Can you work these out from the model? Positions are in its coordinate system, mm. A direction names the side the tool comes from. Coordinates: 2 decimals unless noted, no trailing zeros. Loops run counter-clockwise (first coordinate to the right, second up) from the corner with the lowest first, then second, coordinate; pieces in that order, holes last.
```python
from build123d import *

# Parameters (mm, degrees)
F2_R     = 1.5875
F3_DEPTH = 11.1125
F4_R     = 4.7625
F5_DEPTH = 9.525


with BuildPart() as f1:
    # F0 (on Front) → F1 (revolve)
    with BuildSketch(Plane.XZ):
        with BuildLine():
            Line((0, 63.5), (0, 0))
            Line((0, 0), (5.658861, 0))
            Line((5.658861, 0), (8.89, 5.187289))
            Line((8.89, 5.187289), (25.4, 5.187289))
            ThreePointArc((25.4, 5.187289), (29.890128, 7.047161), (31.75, 11.537289))
            Line((31.75, 11.537289), (31.75, 12.7))
            ThreePointArc((31.75, 12.7), (29.890128, 17.190128), (25.4, 19.05))
            Line((25.4, 19.05), (8.89, 19.05))
            Line((8.89, 19.05), (8.89, 63.5))
            Line((8.89, 63.5), (0, 63.5))
        make_face()
    revolve(axis=Axis((0, 0, 31.75), (0, 0, -1)))

    # F2 (on face) → F3 (cut)
    with BuildSketch(Plane(origin=(0, 0, 0), x_dir=(1, 0, 0), z_dir=(0, 0, -1))):
        Circle(F2_R)
    extrude(amount=-F3_DEPTH, mode=Mode.SUBTRACT)

    # F4 (on face) → F5 (cut)
    with BuildSketch(Plane.XY.offset(63.5)):
        Circle(F4_R)
    extrude(amount=-F5_DEPTH, mode=Mode.SUBTRACT)


solid = f1.part
```
Item 1: On a 3-axis mill with a long thin cutter (end or side, diameter ignored), from which of +Z, -Z, +X, -X, +Y, -Y can I reach the whole of each face in a straight line? I mean faces 5 (the face through (-11, 0, 5.187)), 6 (the face through (-1.2, -1.3, 0)), 7 (the face through (-1.93, 8.68, 41.59)). Say none if no direction works.
Results are:
face 5: -Z
face 6: -Z, +X, -X, +Y, -Y
face 7: +Z
Item 2: Suppose I cut it at C-C, the plane z = 58.5. Please give me the cut outline in (x, y) (1 decimal).
Results are:
outline: circle Ø17.8 at (0, 0); hole circle Ø9.5 at (0, 0)
Item 3: We'd pull the mould along X, two halves only. Please class faces 1 (the face through (-1.3, 5.7, 0.3)), 2 (the face through (-3.78, -2.9, 58.8)), 3 (the face through (0, 0, 11.112)), 4 (the face through (11, 0, 19.05)): +X half, -X half, draft (parallel to the pull), parting line (faces both ways), or undercut.
Results are:
face 1: parting line
face 2: undercut
face 3: undercut
face 4: draft
Item 4: I need wall thicknesses on line 1 along Y through (x, z) = (0, 61.25); line 2 along Z through (x, y) = (21, 3.5); line 3 along Y through (x, z) = (0, 4.75). Which ranges of each line are inside material? Lowest first, please.
Results are:
line 1: y = -8.89 to -4.76, 4.76 to 8.89
line 2: z = 5.19 to 19.05
line 3: y = -8.62 to -1.59, 1.59 to 8.62
Item 5: Suppose I cut it at D-D, the plane z = 35.5. Please give me the cut outline in (x, y).
Results are:
outline: circle Ø17.78 at (0, 0)
Item 6: I'm going to push flat-ended pins straight in: P1, Ø1, axis at x = 0.5, y = 0, coming from the -Z side; P2, Ø5.5, axis at x = 0, y = 0, coming from the +Z side (3 decimals); P3, Ø10, axis at x = -15, z = 12, coming from the -Y side. Where does each tip first touch, or does it pass through?
Results are:
P1: stops at z = 11.11
P2: stops at z = 53.975
P3: stops at y = -30.13
